Geometry: final body of the model. Coordinates: model frame, mm. A direction names the side the tool comes from. Give positions to 0.01 mm unless a question says otherwise; leave off trailing zeros. Order: outer loops, then holes, each group sorted by start corner. A loop starts at its lowest first (then second) coordinate and runs counter-clockwise, first axis right, second up. Notation, with made-up numbers: (-14, 79) -> (8, 79) arc R20 ccw to (8, 109) -> close; hole circle Ø7 at (-35, 76). An arc over 180 degrees is marked (long way). One line per question, with ' | ' between items. Start each with the question number.
(1) Mould query, pull axis X, two halves, no side actions, for faces 3 (the face through (9.4, 4.96, 9.43)), 4 (the face through (3.61, 3.94, 7.54)), 5 (the face through (3.937, 2.956, 2.465)), 6 (the face through (0.57, 0.6, 4.06)). Classes: +X half, -X half, draft (parallel to the pull), parting line (faces both ways), or undercut.
(2) Ray query, L1, parallel to Y at x = 5, z = 6.3; L2, parallel to Y at x = 5, z = 1.45; L3, parallel to Z at x = 6.25, y = 6.75. Return the intervals inside material, ascending.
(3) Section A-A (z = 2.5). Return loops of the section in (x, y).
(4) Set-up query: faces 1 (the face through (0, 5, 4)), 2 (the face through (5, 7, 5)). Return all of +Z, -Z, +X, -X, +Y, -Y with unobstructed straight access to the full face (end or side cutting, diameter ignored); none if empty.
(5) Section D-D (z = 5.25). Return loops of the section in (x, y).
(6) Section B-B (y = 5). Return loops of the section in (x, z).
(7) First-contact query: pin 1 Ø4 at (x, y) = (5, 5) entering from -Z; pin 2 Ø3 at (x, y) = (5, 5) entering from +Z. Flat tips, straight axial feed; report the tip coordinate or a pass-through.
```python
from build123d import *

# Parameters (mm, degrees)
SKETCH1_W           = 10
SKETCH1_H           = 10
BOSS_EXTRUDE1_DEPTH = 10
SKETCH2_R           = 1.75
CUT_EXTRUDE1_DEPTH  = 11
SKETCH3_R           = 2.304
CUT_EXTRUDE2_DEPTH  = 5
FILLET1_R           = 2
FILLET2_R           = 2


with BuildPart() as part:
    # Sketch1 → Boss-Extrude1 (new body)
    with BuildSketch(Plane.XY):
        with Locations((5, 5)):
            Rectangle(SKETCH1_W, SKETCH1_H)
    extrude(amount=BOSS_EXTRUDE1_DEPTH)

    # Sketch2 → Cut-Extrude1 (cut, through all)
    with BuildSketch(Plane.XY.offset(10)):
        with Locations((5, 5)):
            Circle(SKETCH2_R)
    extrude(amount=-CUT_EXTRUDE1_DEPTH, mode=Mode.SUBTRACT)

    # Sketch3 → Cut-Extrude2 (cut)
    with BuildSketch(Plane(origin=(0, 0, 0), x_dir=(-1, 0, 0), z_dir=(0, 0, -1))):
        with Locations((-5, 5)):
            Circle(SKETCH3_R)
    extrude(amount=-CUT_EXTRUDE2_DEPTH, mode=Mode.SUBTRACT)

    # Fillet1
    fillet1_edges = [part.edges().sort_by_distance(p)[0] for p in [
        (0, 10, 5),
        (10, 10, 5),
        (10, 0, 5),
        (0, 0, 5),
    ]]
    fillet(fillet1_edges, radius=FILLET1_R)

    # Fillet2
    fillet2_edges = [part.edges().sort_by_distance(p)[0] for p in [
        (5, 10, 10),
        (10, 5, 10),
        (0, 5, 10),
        (5, 0, 10),
        (9.414213562, 0.585786438, 10),
        (0.585786438, 0.585786438, 10),
        (0.585786438, 9.414213562, 10),
        (9.414213562, 9.414213562, 10),
    ]]
    fillet(fillet2_edges, radius=FILLET2_R)


solid = part.part
```
Response:
1) face 3: +X half | face 4: undercut | face 5: undercut | face 6: -X half
2) L1: y = 0 to 3.25, 6.75 to 10 | L2: y = 0 to 2.7, 7.3 to 10 | L3: z = 5 to 10
3) outline: (0, 2) arc R2 ccw to (2, 0) -> (8, 0) arc R2 ccw to (10, 2) -> (10, 8) arc R2 ccw to (8, 10) -> (2, 10) arc R2 ccw to (0, 8) -> close; hole circle Ø4.61 at (5, 5)
4) face 1: +Z, -Z, -X, +Y, -Y | face 2: -Z
5) outline: (0, 2) arc R2 ccw to (2, 0) -> (8, 0) arc R2 ccw to (10, 2) -> (10, 8) arc R2 ccw to (8, 10) -> (2, 10) arc R2 ccw to (0, 8) -> close; hole circle Ø3.5 at (5, 5)
6) outline: (0, 0) -> (2.7, 0) -> (2.7, 5) -> (3.25, 5) -> (3.25, 10) -> (2, 10) arc R2 ccw to (0, 8) -> close; (6.75, 5) -> (7.3, 5) -> (7.3, 0) -> (10, 0) -> (10, 8) arc R2 ccw to (8, 10) -> (6.75, 10) -> close
7) pin 1: stops at z = 5 | pin 2: passes through
